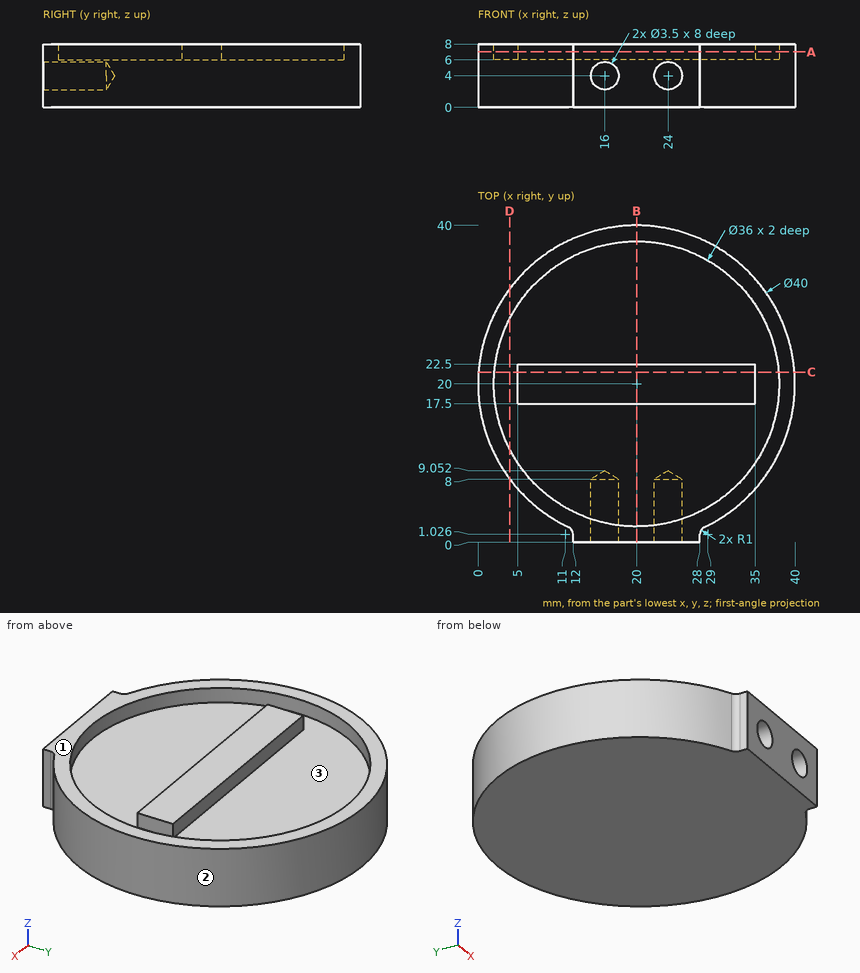
Verification items for this drawing (mm, ordinates from the low corner). Give positions to 0.01 mm unless a question says otherwise; leave off trailing zeros. Loops run counter-clockwise (first coordinate to the right, second up) from the corner with the lowest first, then second, coordinate; pieces in that order, holes last. Notation, with made-up numbers: M 41,28.5 L 96,28.5 A11 ccw 96,44.5 Z; hole C 49,85.25 d3. An arc over 180 degrees is marked long. Answer as a JSON object with one key per item and string values. Group by question number.
Item 1: Sectioned sample at B-B on x = 20. Record the boundary of the cut face in (y, z).
Item 2: Mould release check, pull along X, two halves, no side actions. Record for the marked faces 1, 2 and 3: pulls with the +X half, pulls with the -X half, needs draft (parallel to the pull), parting line crosses it, or undercut.
Item 3: Sectioned sample at A-A on z = 7. Record the boundary of the cut face in (x, y).
Item 4: Sectioned sample at D-D on x = 4. Record the boundary of the cut face in (y, z).
Item 5: Material ranges on L1, parallel to X at y = 20, z = 7; L2, parallel to Y at x = 20, z = 7.4; L3, parallel to Z at x = 16, y = 5, recorded low to high.
Item 6: Sectioned sample at C-C on y = 21.5. Record the boundary of the cut face in (x, z), plus the area to 3 significant figures.
Item 7: Gauge pin test, flat ends, axial feed: pin 1 (2 mm diameter, centred on x = 36, y = 10.5, fed in from -Z); pin 2 (2 mm diameter, centred on y = 19, z = 7, fed in from -X); pin 3 (0.5 mm diameter, centred on y = 0.5, z = 3.5, fed in from +X); pin 4 (0.6 mm diameter, centred on x = 16.5, z = 6.5, fed in from +Y). Record the tip position at first contact, or that the pin passes through.
Findings below:
{
 "1": {"outline": "M 0,0 L 40,0 L 40,8 L 38,8 L 38,6 L 22.5,6 L 22.5,8 L 17.5,8 L 17.5,6 L 2,6 L 2,8 L 0,8 Z"},
 "2": {"face 1": "needs draft", "face 2": "parting line crosses it", "face 3": "undercut"},
 "3": {"outline": "M 5,17.5 L 35,17.5 L 35,22.5 L 5,22.5 Z; M 11.43,1.93 A1 cw 12,1.03 L 12,0 L 28,0 L 28,1.03 A1 cw 28.57,1.93 A20 ccw long Z; hole C 20,20 d36"},
 "4": {"outline": "M 8,0 L 32,0 L 32,8 L 28.25,8 L 28.25,6 L 11.75,6 L 11.75,8 L 8,8 Z"},
 "5": {"L1": "0 to 2, 5 to 35, 38 to 40", "L2": "0 to 2, 17.5 to 22.5, 38 to 40", "L3": "0 to 2.25, 5.75 to 6"},
 "6": {"outline": "M 0.06,0 L 39.94,0 L 39.94,8 L 37.94,8 L 37.94,6 L 35,6 L 35,8 L 5,8 L 5,6 L 2.06,6 L 2.06,8 L 0.06,8 Z", "area": "307 mm2"},
 "7": {"pin 1": "z = 0", "pin 2": "x = 0", "pin 3": "x = 28", "pin 4": "y = 39.74"}
}
